```python
from build123d import *

# Parameters (mm, degrees)
ESQUISSE1_R      = 20
ESQUISSE1_R_2    = 9
ESQUISSE1_R_3    = 1.5
EXTRUSION1_DEPTH = 4
CHANFREIN1_SIZE  = 2
CHANFREIN2_SIZE  = 0.5


with BuildPart() as part:
    # Esquisse1 → Extrusion1 (new body)
    with BuildSketch(Plane.XY):
        Circle(ESQUISSE1_R)
        Circle(ESQUISSE1_R_2, mode=Mode.SUBTRACT)
        with Locations((0, 14)):
            Circle(ESQUISSE1_R_3, mode=Mode.SUBTRACT)
        with Locations((-14, 0)):
            Circle(ESQUISSE1_R_3, mode=Mode.SUBTRACT)
        with Locations((14, 0)):
            Circle(ESQUISSE1_R_3, mode=Mode.SUBTRACT)
        with Locations((0, -14)):
            Circle(ESQUISSE1_R_3, mode=Mode.SUBTRACT)
    extrude(amount=EXTRUSION1_DEPTH)

    # Chanfrein1
    chanfrein1_edges = [part.edges().sort_by_distance(p)[0] for p in [
        (-15.5, 0, 4),
        (12.5, 0, 4),
        (-1.5, -14, 4),
        (-1.5, 14, 4),
    ]]
    chamfer(chanfrein1_edges, length=CHANFREIN1_SIZE)

    # Chanfrein2
    chanfrein2_edges = [part.edges().sort_by_distance(p)[0] for p in [
        (-20, 0, 0),
        (-20, 0, 4),
        (-9, 0, 0),
        (-9, 0, 4),
    ]]
    chamfer(chanfrein2_edges, length=CHANFREIN2_SIZE)


solid = part.part
```
For this review, take the finished solid that the model builds, in its own axes (mm). Coordinates: 2 decimals unless noted, no trailing zeros. Write each loop counter-clockwise with the first axis right and the second up, starting at its lowest first coordinate (ties: lowest second). Pieces come first, ordered by that corner, then holes. Notation, with made-up numbers: (9, 82.25) - (40, 82.25) arc R19 ccw to (40, 88.25) - close; hole circle Ø9 at (-39.5, -17.75). An arc over 180 degrees is marked (long way). Answer in a Markdown table with one row per item. Add a question column.
Q1. We need section B-B, the plane z = 1.5. State the section outline as (x, y) points, and give its area (3 significant figures).
Q2. Draft analysis for pull direction Y (two halves, no side actions). For faces 1 (the cylindrical face through (-4.336, -19.524, 1.979)), 2 (the conical face through (-15.624, 0.071, 2.125)), 3 (the flat face through (4, 9, 0)), state which applies: +Y half, -Y half, draft (parallel to the pull), parting line (faces both ways), or undercut.
Q3. For P1, Ø6, axis at x = -3, y = -13, coming from the -Z side; P2, Ø2, axis at y = 13.5, z = 2, coming from the -X side; P3, Ø2, axis at x = -3, z = 3, coming from the -Y side; P4, Ø5, axis at x = 0, y = 14, coming from the +Z side, all flat-tipped, find the tip position at first contact; note any pin that passes through.
Q4. For probe 1 along Y at (x, z) = (-13, 3.4); probe 2 along X at (y, z) = (-2.5, 1.8); probe 3 along X at (y, z) = (6.5, 2.7), list the stretches that pass through material, from the lowest coordinate up.
Q5. We need section A-A, the plane x = 0. State the section outline as (y, z) points, and give its area (3 significant figures).
Answer list:
| question | item | result |
|---|---|---|
| 1 | outline | circle Ø40 at (0, 0); hole circle Ø3 at (-14, 0); hole circle Ø18 at (0, 0); hole circle Ø3 at (0, -14); hole circle Ø3 at (0, 14); hole circle Ø3 at (14, 0) |
| 1 | area | 974 mm2 |
| 2 | face 1 | parting line |
| 2 | face 2 | undercut |
| 2 | face 3 | draft |
| 3 | P1 | stops at z = 0 |
| 3 | P2 | stops at x = -15.61 |
| 3 | P3 | stops at y = -19.9 |
| 3 | P4 | stops at z = 3 |
| 4 | probe 1 | y = -15.2 to -2.72, 2.72 to 15.2 |
| 4 | probe 2 | x = -19.84 to -8.65, 8.65 to 19.84 |
| 4 | probe 3 | x = -18.91 to -6.22, 6.22 to 18.91 |
| 5 | outline | (-20, 0.5) - (-19.5, 0) - (-15.5, 0) - (-15.5, 2) - (-17.5, 4) - (-19.5, 4) - (-20, 3.5) - close; (-12.5, 0) - (-9.5, 0) - (-9, 0.5) - (-9, 3.5) - (-9.5, 4) - (-10.5, 4) - (-12.5, 2) - close; (9, 0.5) - (9.5, 0) - (12.5, 0) - (12.5, 2) - (10.5, 4) - (9.5, 4) - (9, 3.5) - close; (15.5, 0) - (19.5, 0) - (20, 0.5) - (20, 3.5) - (19.5, 4) - (17.5, 4) - (15.5, 2) - close |
| 5 | area | 55.0 mm2 |
